CAD build for the part. Positions are in the model's coordinates, mm. A direction names the side the tool comes from. Round coordinates to 2 decimals unless told otherwise and drop trailing zeros. Write each loop counter-clockwise with the first axis right and the second up, starting at its lowest first coordinate (ties: lowest second). Pieces come first, ordered by that corner, then holes. Notation, with made-up numbers: (9, 76.25) -> (57, 76.25) arc R15 cw to (57, 83.25) -> close; hole circle Ø2 at (-6, 65.25). An arc over 180 degrees is marked (long way). Answer in a Markdown table with one row per item. Add a question column.
Autodesk Inventor part; units mm, degrees
ref_plane "YZ Plane" through (0, 0, 0) normal (1, 0, 0) x (0, 1, 0)
ref_plane "XZ Plane" through (0, 0, 0) normal (0, 1, 0) x (-1, 0, 0)
ref_plane "XY Plane" through (0, 0, 0) normal (0, 0, 1) x (1, 0, 0)
sketch "Sketch1" plane through (0, 0, 0) normal (1, 0, 0) x (0, 1, 0)
  line L0 (25.0368, -4.28) -> (3.9428, -127.674)
  arc A0 (-4, -127) -> (3.9428, -127.674) centre (0, -127) ccw
  arc A1 (25.0368, -4.28) -> (-16.84, -19.0151) centre (0, 0) ccw
  line L1 (0, 0) -> (0, -127) construction
  circle A2 centre (0, 0) radius 16
  circle A3 centre (0, -127) radius 2
  circle A4 centre (0, -63.5) radius 2
  line L2 (-4, -127) -> (-4, -47.5378)
  arc A5 (-4, -47.5378) -> (-16.84, -19.0151) centre (-42.1, -47.5378) ccw
  dimension "d0" = 32
  dimension "d1" = 127
  dimension "d2" = 4
  dimension "d3" = 25.4
  dimension "d4" = 4
  dimension "d7" = 63.5
  dimension "d14" = 38.1
extrude "Extrusion1" add sketch "Sketch1" along normal blind 3
properties part number "linkPanel" material "CFRP"
Item 1: Saw through at C-C on x = 0.5. Give the cut face in (y, z), then the cut area to 3 significant figures.
Item 2: Tool access for faces 4 (the cylindrical face through (1, 0, -129)), 5 (the flat face through (1, -4, -88)): list every direction of +Z, -Z, +X, -X, +Y, -Y with a clear straight run to the whole face (end or side of a thin tool).
Item 3: Saw through at D-D on y = 12. Give the cut face in (x, z), then the cut area to 3 significant figures.
Item 4: Saw through at B-B on y = 0. Give the cut face in (x, z).
Item 5: Saw through at A-A on z = 0. Give the cut face in (x, y), then the cut area to 3 significant figures.
Item 6: Two-plate mould, pull along Z, no slides. Class faces 1 (the flat face through (0, 5, -34)), 2 (the cylindrical face through (1.48, -3.47, 15.62)), 3 (the cylindrical face through (1.479, -9.124, 23.705)): +Z half, -Z half, draft (parallel to the pull), parting line (faces both ways), or undercut.
Item 7: Pin check, flat tips, straight feed: pin 1 (3.5 mm diameter, centred on y = 0, z = -63.5, fed in from +X); pin 2 (1.5 mm diameter, centred on x = 1, z = -93.5, fed in from -Y); pin 3 (1.5 mm diameter, centred on x = 0.5, y = -12.5, fed in from -Z). Stop position of each tip, or through.
Item 8: Drill centre lines: probe 1 along Z at (x, y) = (1.4, 0); probe 2 along Z at (x, y) = (0.5, -3.5); probe 3 along Z at (x, y) = (1.5, -10). Where is each one in solid material? Low to high.
Recorded:
| question | item | result |
|---|---|---|
| 1 | outline | (-16.84, -19.02) arc R38.1 cw to (-4, -47.54) -> (-4, -127) arc R4 ccw to (3.94, -127.67) -> (25.04, -4.28) arc R25.4 ccw (long way) to start; hole circle Ø32 at (0, 0); hole circle Ø4 at (0, -127); hole circle Ø4 at (0, -63.5) |
| 1 | area | 3,080 mm2 |
| 2 | face 4 | +X, -X |
| 2 | face 5 | -Z, +X, -X, -Y |
| 3 | outline | (0, -80.54) -> (3, -80.54) -> (3, -10.58) -> (0, -10.58) -> close; (0, 10.58) -> (3, 10.58) -> (3, 22.39) -> (0, 22.39) -> close |
| 3 | area | 245 mm2 |
| 4 | outline | (0, -131) -> (3, -131) -> (3, -129) -> (0, -129) -> close; (0, -125) -> (3, -125) -> (3, -65.5) -> (0, -65.5) -> close; (0, -61.5) -> (3, -61.5) -> (3, -16) -> (0, -16) -> close; (0, 16) -> (3, 16) -> (3, 25.4) -> (0, 25.4) -> close |
| 5 | outline | (0, -25.4) -> (3, -25.4) -> (3, -16) -> (0, -16) -> close; (0, 16) -> (3, 16) -> (3, 25.4) -> (0, 25.4) -> close |
| 5 | area | 56.4 mm2 |
| 6 | face 1 | draft |
| 6 | face 2 | undercut |
| 6 | face 3 | parting line |
| 7 | pin 1 | through |
| 7 | pin 2 | y = -4 |
| 7 | pin 3 | z = -24.51 |
| 8 | probe 1 | -131 to -129, -125 to -65.5, -61.5 to -16, 16 to 25.4 |
| 8 | probe 2 | -128.94 to -15.61, 15.61 to 25.16 |
| 8 | probe 3 | -27.01 to -12.49, 12.49 to 23.35 |
